Model file for the job. Use its own axes, mm. Face numbers are marked on the shaded views. A direction names the side the tool comes from. Coordinates: 2 decimals unless noted, no trailing zeros. Write each loop counter-clockwise with the first axis right and the second up, starting at its lowest first coordinate (ties: lowest second). Pieces come first, ordered by that corner, then holes. Notation, with made-up numbers: M 13.5,61 L 40.5,61 A31 ccw 40.5,93 Z; hole C 49,-4 d8. An arc over 180 degrees is marked long. Put each result on its own line as item: value. Start each with the question number.
Q1. Cut at B-B (y = -32). Give the number of separate pieces and of enclosed holes in the cut face, then the cut area to 3 significant figures.
Q2. Cut at D-D (z = -2). Write the cut outline in (x, y), then the cut area to 4 significant figures.
Q3. Drop flat-ended pins along their axis: pin 1 (4 mm diameter, centred on x = -6, y = 0, fed in from -Z); pin 2 (1.6 mm diameter, centred on x = -1, y = -5, fed in from +Z); pin 3 (6.5 mm diameter, centred on x = 4.24, y = -4.24, fed in from -Z); pin 4 (5 mm diameter, centred on x = -27.5, y = -27.5, fed in from +Z). Give the stop position or say it passes through.
Q4. Cut at C-C (x = -38). Write the cut outline in (y, z).
Q5. Cut at A-A (z = -17). Write the cut outline in (x, y), then the cut area to 3 significant figures.
Q6. Pull direction Z, two halves, no side cores. Call the marked faces 1, 2 and 3: pulls with the +Z half, pulls with the -Z half, needs draft (parallel to the pull), parting line crosses it, or undercut.
Q7. Drill centre lines: line 1 along Z through (x, y) = (-25, -21.5); line 2 along X through (y, z) = (-22.5, -10); line 3 along Z through (x, y) = (-13, -11). Where is each one in solid material? Low to high.
Q8. Which spindle directions (+Z, -Z, +X, -X, +Y, -Y) get a long thin tool onto all of the face, cutting with end or side? Do the marked faces 4, 5, 6, 7 and 8. Say none if no direction does.
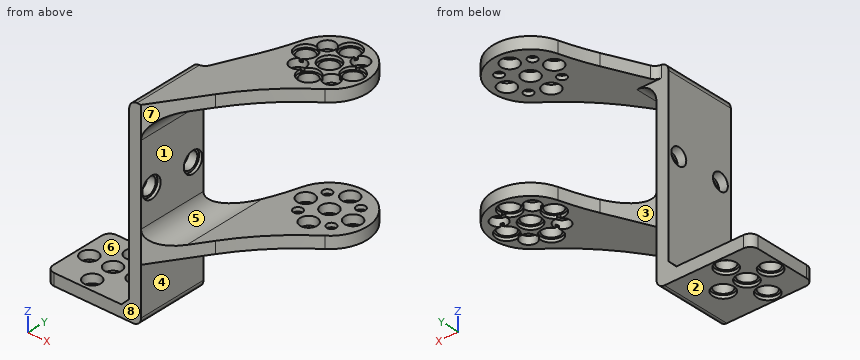
```python
from build123d import *

# Parameters (mm, degrees)
SKETCH1_R                                            = 2
BOSS_EXTRUDE1_DEPTH                                  = 3
SKETCH23_R                                           = 2.15
CUT_EXTRUDE5_DEPTH                                   = 41.422765863
SKETCH2_W                                            = 3
SKETCH2_H                                            = 18
BOSS_EXTRUDE2_DEPTH                                  = 44
SKETCH3_R                                            = 2.15
BOSS_EXTRUDE3_DEPTH                                  = 3
SKETCH5_R                                            = 2.65
CUT_EXTRUDE1_DEPTH                                   = 0.8
CUT_EXTRUDE2_START                                   = -0.8
SKETCH11_R                                           = 2.65
CUT_EXTRUDE2_DEPTH                                   = 0.8
SKETCH12_W                                           = 24
SKETCH12_H                                           = 18
SKETCH12_R                                           = 2
BOSS_EXTRUDE4_DEPTH                                  = 3
SKETCH24_R                                           = 2.15
CUT_EXTRUDE6_DEPTH                                   = 74.525505779
HOLE1_D                                              = 4.3
HOLE1_CBORE_D                                        = 5.3
HOLE1_CBORE_DEPTH                                    = 0.8
SKETCH22_R                                           = 2.65
CUT_EXTRUDE4_DEPTH                                   = 0.8
CBORE_FOR_M1_6_HEX_SOCKET_HEAD_CAP_SCREW_D           = 2.3
CBORE_FOR_M1_6_HEX_SOCKET_HEAD_CAP_SCREW_DEPTH       = 3
CBORE_FOR_M1_6_HEX_SOCKET_HEAD_CAP_SCREW_CBORE_D     = 4
CBORE_FOR_M1_6_HEX_SOCKET_HEAD_CAP_SCREW_CBORE_DEPTH = 2
CBORE_FOR_M1_6_HEX_SOCKET_HEAD_CAP_S_2_D             = 2.3
CBORE_FOR_M1_6_HEX_SOCKET_HEAD_CAP_S_2_CBORE_D       = 4
CBORE_FOR_M1_6_HEX_SOCKET_HEAD_CAP_S_2_CBORE_DEPTH   = 2
HOLE2_D                                              = 4.3
HOLE2_DEPTH                                          = 3
HOLE2_CBORE_D                                        = 5.3
HOLE2_CBORE_DEPTH                                    = 0.8
HOLE3_D                                              = 4.3
HOLE3_CBORE_D                                        = 5.3
HOLE3_CBORE_DEPTH                                    = 0.8
FILLET10_R                                           = 2
FILLET5_R                                            = 2
CHAMFER2_SIZE                                        = 2
FILLET7_R                                            = 60
REDONDEO1_R                                          = 5


with BuildPart() as part:
    # Sketch1 → Boss-Extrude1 (new body)
    with BuildSketch(Plane.XY):
        with BuildLine():
            Line((0, -9.5), (-17, -35))
            Line((-17, -35), (-20, -35))
            Line((-20, -35), (-20, -17))
            Line((-20, -17), (-17, -17))
            Line((-17, -17), (-9.5, 0))
            ThreePointArc((-9.5, 0), (6.717514421, 6.717514421), (0, -9.5))
        make_face()
        with Locations((-6, 0)):
            Circle(SKETCH1_R, mode=Mode.SUBTRACT)
        with Locations((0, -6)):
            Circle(SKETCH1_R, mode=Mode.SUBTRACT)
        with Locations((6, 0)):
            Circle(SKETCH1_R, mode=Mode.SUBTRACT)
        with Locations((0, 6)):
            Circle(SKETCH1_R, mode=Mode.SUBTRACT)
    extrude(amount=BOSS_EXTRUDE1_DEPTH)

    # Sketch23 → Cut-Extrude5 (cut, through all)
    with BuildSketch(Plane.XY.offset(3)):
        with Locations((6, 0)):
            Circle(SKETCH23_R)
        with Locations((0, -6)):
            Circle(SKETCH23_R)
        with Locations((-6, 0)):
            Circle(SKETCH23_R)
        with Locations((0, 6)):
            Circle(SKETCH23_R)
    extrude(amount=-CUT_EXTRUDE5_DEPTH, mode=Mode.SUBTRACT)

    # Sketch2 → Boss-Extrude2 (add)
    with BuildSketch(Plane(origin=(0, 0, 0), x_dir=(-1, 0, 0), z_dir=(0, 0, -1))):
        with Locations((18.5, -26)):
            Rectangle(SKETCH2_W, SKETCH2_H)
    extrude(amount=BOSS_EXTRUDE2_DEPTH)

    # Sketch3 → Boss-Extrude3 (add)
    with BuildSketch(Plane(origin=(0, 0, -30), x_dir=(-1, 0, 0), z_dir=(0, 0, -1))):
        with BuildLine():
            Line((20, -17), (17, -17))
            Line((17, -17), (9.5, 0))
            ThreePointArc((9.5, 0), (-6.717514421, 6.717514421), (0, -9.5))
            Line((0, -9.5), (17, -35))
            Line((17, -35), (20, -35))
            Line((20, -35), (20, -17))
        make_face()
        with Locations(Location((0, -6, 0), (0, 0, 180))):
            Circle(SKETCH3_R, mode=Mode.SUBTRACT)
        with Locations(Location((-6, 0, 0), (0, 0, 180))):
            Circle(SKETCH3_R, mode=Mode.SUBTRACT)
        with Locations(Location((6, 0, 0), (0, 0, 180))):
            Circle(SKETCH3_R, mode=Mode.SUBTRACT)
        with Locations(Location((0, 6, 0), (0, 0, 180))):
            Circle(SKETCH3_R, mode=Mode.SUBTRACT)
    extrude(amount=BOSS_EXTRUDE3_DEPTH)

    # Sketch5 → Cut-Extrude1 (cut)
    with BuildSketch(Plane.XY.offset(3)):
        with Locations((0, -6)):
            Circle(SKETCH5_R)
        with Locations((-6, 0)):
            Circle(SKETCH5_R)
        with Locations((0, 6)):
            Circle(SKETCH5_R)
        with Locations((6, 0)):
            Circle(SKETCH5_R)
    extrude(amount=-CUT_EXTRUDE1_DEPTH, mode=Mode.SUBTRACT)

    # Sketch11 → Cut-Extrude2 (cut)
    with BuildSketch(Plane(origin=(0, 0, -33), x_dir=(-1, 0, 0), z_dir=(0, 0, -1)).offset(CUT_EXTRUDE2_START)):
        with Locations(Location((0, 6, 0), (0, 0, 180))):
            Circle(SKETCH11_R)
        with Locations(Location((-6, 0, 0), (0, 0, 180))):
            Circle(SKETCH11_R)
        with Locations(Location((0, -6, 0), (0, 0, 180))):
            Circle(SKETCH11_R)
        with Locations(Location((6, 0, 0), (0, 0, 180))):
            Circle(SKETCH11_R)
    extrude(amount=CUT_EXTRUDE2_DEPTH, mode=Mode.SUBTRACT)

    # Sketch12 → Boss-Extrude4 (add)
    with BuildSketch(Plane(origin=(0, 0, -44), x_dir=(-1, 0, 0), z_dir=(0, 0, -1))):
        with Locations((29, -26)):
            Rectangle(SKETCH12_W, SKETCH12_H)
        with Locations((38, -26)):
            Circle(SKETCH12_R, mode=Mode.SUBTRACT)
        with Locations((32, -32)):
            Circle(SKETCH12_R, mode=Mode.SUBTRACT)
        with Locations((32, -26)):
            Circle(SKETCH12_R, mode=Mode.SUBTRACT)
        with Locations((32, -20)):
            Circle(SKETCH12_R, mode=Mode.SUBTRACT)
        with Locations((26, -26)):
            Circle(SKETCH12_R, mode=Mode.SUBTRACT)
    extrude(amount=BOSS_EXTRUDE4_DEPTH)

    # Sketch24 → Cut-Extrude6 (cut, through all)
    with BuildSketch(Plane(origin=(0, 0, -47), x_dir=(-1, 0, 0), z_dir=(0, 0, -1))):
        with Locations((32, -20)):
            Circle(SKETCH24_R)
        with Locations((26, -26)):
            Circle(SKETCH24_R)
        with Locations((32, -26)):
            Circle(SKETCH24_R)
        with Locations((38, -26)):
            Circle(SKETCH24_R)
        with Locations((32, -32)):
            Circle(SKETCH24_R)
    extrude(amount=-CUT_EXTRUDE6_DEPTH, mode=Mode.SUBTRACT)

    # Hole1 (through all)
    with Locations(Plane(origin=(-17, 0, 0), x_dir=(0, 0, -1), z_dir=(1, 0, 0))):
        with Locations((17, -20), (17, -32)):
            CounterBoreHole(HOLE1_D / 2, HOLE1_CBORE_D / 2, HOLE1_CBORE_DEPTH)

    # Sketch22 → Cut-Extrude4 (cut)
    with BuildSketch(Plane(origin=(0, 0, -47), x_dir=(-1, 0, 0), z_dir=(0, 0, -1))):
        with Locations((32, -32)):
            Circle(SKETCH22_R)
        with Locations((38, -26)):
            Circle(SKETCH22_R)
        with Locations((32, -26)):
            Circle(SKETCH22_R)
        with Locations((32, -20)):
            Circle(SKETCH22_R)
        with Locations((26, -26)):
            Circle(SKETCH22_R)
    extrude(amount=-CUT_EXTRUDE4_DEPTH, mode=Mode.SUBTRACT)

    # CBORE for M1.6 Hex Socket Head Cap Screw
    with Locations(Plane.XY.offset(3)):
        with Locations((-4.242640687, -4.242640687), (4.242640687, -4.242640687), (4.242640687, 4.242640687), (-4.242640687, 4.242640687)):
            CounterBoreHole(CBORE_FOR_M1_6_HEX_SOCKET_HEAD_CAP_SCREW_D / 2, CBORE_FOR_M1_6_HEX_SOCKET_HEAD_CAP_SCREW_CBORE_D / 2, CBORE_FOR_M1_6_HEX_SOCKET_HEAD_CAP_SCREW_CBORE_DEPTH, depth=CBORE_FOR_M1_6_HEX_SOCKET_HEAD_CAP_SCREW_DEPTH)

    # CBORE for M1.6 Hex Socket Head Cap S 2 (through all)
    with Locations(Plane(origin=(0, 0, -33), x_dir=(-1, 0, 0), z_dir=(0, 0, -1))):
        with Locations((4.242640687, 4.242640687), (4.242640687, -4.242640687), (-4.242640687, -4.242640687), (-4.242640687, 4.242640687)):
            CounterBoreHole(CBORE_FOR_M1_6_HEX_SOCKET_HEAD_CAP_S_2_D / 2, CBORE_FOR_M1_6_HEX_SOCKET_HEAD_CAP_S_2_CBORE_D / 2, CBORE_FOR_M1_6_HEX_SOCKET_HEAD_CAP_S_2_CBORE_DEPTH)

    # Hole2
    with Locations(Plane.XY.offset(3)):
        with Locations((0, 0)):
            CounterBoreHole(HOLE2_D / 2, HOLE2_CBORE_D / 2, HOLE2_CBORE_DEPTH, depth=HOLE2_DEPTH)

    # Hole3 (through all)
    with Locations(Plane(origin=(0, 0, -33), x_dir=(-1, 0, 0), z_dir=(0, 0, -1))):
        with Locations((0, 0)):
            CounterBoreHole(HOLE3_D / 2, HOLE3_CBORE_D / 2, HOLE3_CBORE_DEPTH)

    # Fillet10
    fillet10_edges = [part.edges().sort_by_distance(p)[0] for p in [
        (-17, -17, 1.5),
    ]]
    fillet(fillet10_edges, radius=FILLET10_R)

    # Fillet5
    fillet5_edges = [part.edges().sort_by_distance(p)[0] for p in [
        (-41, -17, -45.5),
        (-41, -35, -45.5),
        (-17, -26, -47),
        (-20, -26, 3),
    ]]
    fillet(fillet5_edges, radius=FILLET5_R)

    # Chamfer2
    chamfer2_edges = [part.edges().sort_by_distance(p)[0] for p in [
        (-20, -26, -44),
    ]]
    chamfer(chamfer2_edges, length=CHAMFER2_SIZE)

    # Fillet7
    fillet7_edges = [part.edges().sort_by_distance(p)[0] for p in [
        (0, -9.5, 1.5),
        (-9.5, 0, 1.5),
        (-9.5, 0, -31.5),
        (0, -9.5, -31.5),
    ]]
    fillet(fillet7_edges, radius=FILLET7_R)

    # Redondeo1
    # the kernel refuses this fillet: 5 mm, written as the material it adds along each edge
    with BuildSketch(Plane(origin=(-17, -47.5, -30), x_dir=(0, 0, 1), z_dir=(0, 1, 0))) as redondeo1_piece_1_section:
        with BuildLine():
            CenterArc((REDONDEO1_R, REDONDEO1_R), REDONDEO1_R, 180, 90)
            Line((0, REDONDEO1_R), (0, 0))
            Line((0, 0), (REDONDEO1_R, 0))
        make_face()
    redondeo1_piece_1 = extrude(amount=43, mode=Mode.PRIVATE)
    redondeo1_piece_1 = split(redondeo1_piece_1, bisect_by=Plane(origin=(-12.168719693, -27.753079539, -28.835648112), z_dir=(-0.8320502943378423, 0.5547001962252313, 0)), keep=Keep.TOP, mode=Mode.PRIVATE)
    redondeo1_piece_1 = split(redondeo1_piece_1, bisect_by=Plane(origin=(-19.867910191, -23.500596432, -28.835648112), z_dir=(0.9149178015729305, -0.40364020657629746, 0)), keep=Keep.TOP, mode=Mode.PRIVATE)
    add(redondeo1_piece_1)
    with BuildSketch(Plane(origin=(-17, -47.5, 0), x_dir=(1, 0, 0), z_dir=(0, 1, 0))) as redondeo1_piece_2_section:
        with BuildLine():
            CenterArc((REDONDEO1_R, REDONDEO1_R), REDONDEO1_R, 180, 90)
            Line((0, REDONDEO1_R), (0, 0))
            Line((0, 0), (REDONDEO1_R, 0))
        make_face()
    redondeo1_piece_2 = extrude(amount=30.5, mode=Mode.PRIVATE)
    redondeo1_piece_2 = split(redondeo1_piece_2, bisect_by=Plane(origin=(-12.168719693, -27.753079539, -1.164351888), z_dir=(-0.8320502943378424, 0.5547001962252313, 0)), keep=Keep.TOP, mode=Mode.PRIVATE)
    add(redondeo1_piece_2)


solid = part.part
```
Computed values:
1. separate pieces: 3
1. enclosed holes: 0
1. area: 207 mm2
2. outline: M -20,-35 L -17,-35 L -16,-33.5 L -16,-17 L -20,-17 Z
2. area: 71.25 mm2
3. pin 1: through
3. pin 2: z = 2.2
3. pin 3: z = -33
3. pin 4: z = -44
4. outline: M -35,-47 L -28.65,-47 L -28.65,-46.2 L -28.15,-46.2 L -28.15,-44 L -35,-44 Z; M -23.85,-46.2 L -23.35,-46.2 L -23.35,-47 L -17,-47 L -17,-44 L -23.85,-44 Z
5. outline: M -20,-35 L -17,-35 L -17,-34.65 L -17.8,-34.65 L -17.8,-34.15 L -20,-34.15 Z; M -20,-29.85 L -17.8,-29.85 L -17.8,-29.35 L -17,-29.35 L -17,-22.65 L -17.8,-22.65 L -17.8,-22.15 L -20,-22.15 Z; M -20,-17.85 L -17.8,-17.85 L -17.8,-17.35 L -17,-17.35 L -17,-17 L -20,-17 Z
5. area: 26.6 mm2
6. face 1: undercut
6. face 2: pulls with the -Z half
6. face 3: needs draft
7. line 1: -47 to -44
7. line 2: -20 to -17
7. line 3: -33 to -29.9, 0 to 3
8. face 4: -Z, +X, +Y, -Y
8. face 5: +X, +Y, -Y
8. face 6: +Z, -X, +Y, -Y
8. face 7: +Z, -Z, +X, -Y
8. face 8: +Z, -Z, +X, -X, -Y
